Drawing for the job (mm, zero at the part's lowest x, y, z). A direction names the side the tool comes from. Coordinates: 2 decimals unless noted, no trailing zeros. Order: outer loops, then holes, each group sorted by start corner. A loop starts at its lowest first (then second) coordinate and runs counter-clockwise, first axis right, second up.
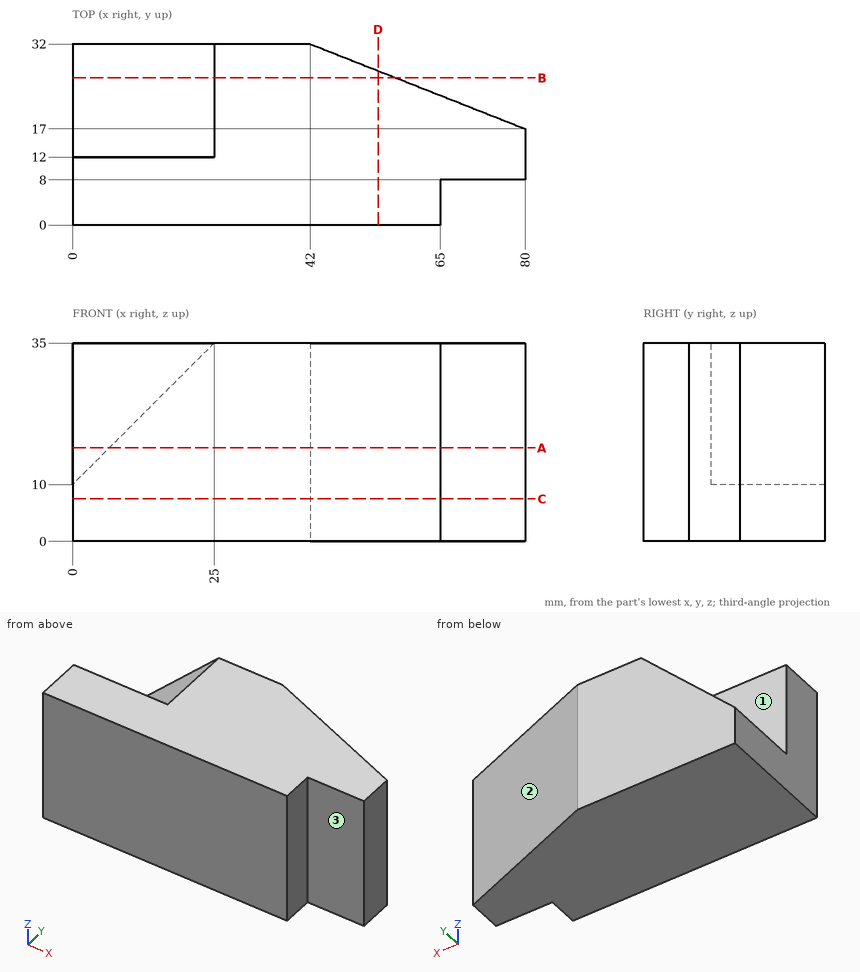
(1) Slice it at B-B, the plane y = 26. Give the cut face in (x, z), then the cut area to 3 significant figures.
(2) Slice it at C-C, the plane z = 7.5. Give the cut face in (x, y), then the cut area to 4 significant figures.
(3) Probe line 1 (X direction, y = 4.5, z = 2.5); line 2 (Y direction, x = 18, z = 30); line 3 (Y direction, x = 49, z = 24). List the from-to ranges inside material, lowest first.
(4) Slice it at A-A, the plane z = 16.5. Give the cut face in (x, y).
(5) Drop a flat-ended pin along its axis: pin 1 (6.5 mm diameter, centred on y = 4, z = 25, fed in from +X). Give the stop position or say it passes through.
(6) Tool access for the marked faces 1, 2 and 3: list every direction of +Z, -Z, +X, -X, +Y, -Y with a clear straight run to the whole face (end or side of a thin tool).
(7) Slice it at D-D, the plane x = 54. Give the cut face in (y, z).
Here are the results:
1. outline: (0, 0) - (57.2, 0) - (57.2, 35) - (25, 35) - (0, 10) - close
1. area: 1,690 mm2
2. outline: (0, 0) - (65, 0) - (65, 8) - (80, 8) - (80, 17) - (42, 32) - (0, 32) - close
2. area: 2,155 mm2
3. line 1: x = 0 to 65
3. line 2: y = 0 to 12
3. line 3: y = 0 to 29.24
4. outline: (0, 0) - (65, 0) - (65, 8) - (80, 8) - (80, 17) - (42, 32) - (6.5, 32) - (6.5, 12) - (0, 12) - close
5. pin 1: stops at x = 65
6. face 1: +Z, -X, +Y
6. face 2: +Z, -Z, +X, +Y
6. face 3: +Z, -Z, +X, -Y
7. outline: (0, 0) - (27.26, 0) - (27.26, 35) - (0, 35) - close
